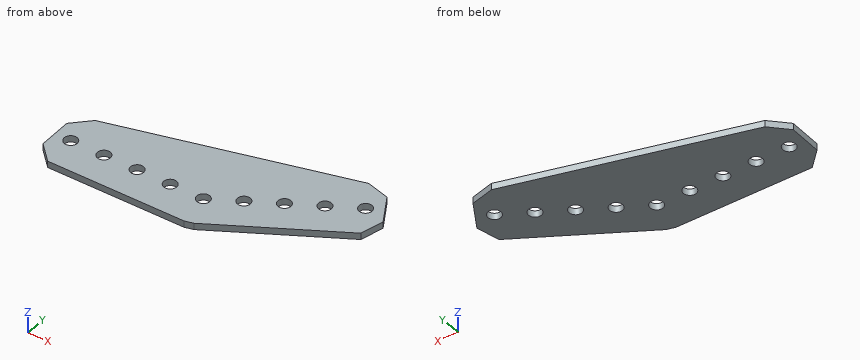
from build123d import *

# Parameters (mm, degrees)
SKETCH1_R           = 2.5
BOSS_EXTRUDE1_DEPTH = 2.5


with BuildPart() as part:
    # Sketch1 → Boss-Extrude1 (new body)
    with BuildSketch(Plane(origin=(0, 0, -1.25), x_dir=(-1, 0, 0), z_dir=(0, 0, -1))):
        Polygon((50.546, 12.7), (-37.42412006, 36.271522628), (-46.098381374, 33.947261314), (-52.448381374, 22.948738686), (-50.12412006, 14.274477372), (-4.902017026, -11.834515988), (-1.671986719, -12.7), (50.546, -12.7), (56.896, -6.35), (56.896, 6.35), align=None)
        with Locations((12.7, 0)):
            Circle(SKETCH1_R, mode=Mode.SUBTRACT)
        with Locations((25.4, 0)):
            Circle(SKETCH1_R, mode=Mode.SUBTRACT)
        Circle(SKETCH1_R, mode=Mode.SUBTRACT)
        with Locations((50.8, 0)):
            Circle(SKETCH1_R, mode=Mode.SUBTRACT)
        with Locations((38.1, 0)):
            Circle(SKETCH1_R, mode=Mode.SUBTRACT)
        with Locations((-43.994090512, 25.4)):
            Circle(SKETCH1_R, mode=Mode.SUBTRACT)
        with Locations((-32.995567884, 19.05)):
            Circle(SKETCH1_R, mode=Mode.SUBTRACT)
        with Locations((-21.997045256, 12.7)):
            Circle(SKETCH1_R, mode=Mode.SUBTRACT)
        with Locations((-10.998522628, 6.35)):
            Circle(SKETCH1_R, mode=Mode.SUBTRACT)
    extrude(amount=-BOSS_EXTRUDE1_DEPTH)


solid = part.part
The model under review builds one solid part; all positions refer to its coordinate system, in mm. Give positions to 0.01 mm unless a question says otherwise; leave off trailing zeros. Write each loop counter-clockwise with the first axis right and the second up, starting at its lowest first coordinate (ties: lowest second). Pieces come first, ordered by that corner, then holes.
1. Add section D-D, the plane y = 19.05. Write out the cut boundary in (x, z), plus the area to 3 significant figures.
2. For P1, Ø4.5, axis at x = 22, y = 12.7, coming from the +Z side, flat-tipped, find the tip position at first contact; note if it passes through.
3. Wall thickness on L1, parallel to Y at x = -12.5, z = 0; L2, parallel to Y at x = -50.8, z = 0.3; L3, parallel to Y at x = -22, z = 0.2: over which ranges is each line inside the solid? List them lowest first.
4. Add section A-A, the plane y = 0. Write out the cut boundary in (x, z).
5. Add section C-C, the plane x = -12.7. Write out the cut boundary in (y, z), plus the area to 3 significant figures.
6. Add section B-B, the plane z = -0.55. Count the separate pieces of the cut face and the enclosed holes in it, plus the area to 3 significant figures.
Worked answers:
1. outline: (-26.85, -1.25) - (30.5, -1.25) - (30.5, 1.25) - (-26.85, 1.25) - close; (35.5, -1.25) - (51.4, -1.25) - (51.4, 1.25) - (35.5, 1.25) - close
1. area: 183 mm2
2. P1: passes through
3. L1: y = -12.7 to -2.49, 2.49 to 22.89
3. L2: y = -12.45 to -2.5, 2.5 to 12.45
3. L3: y = -12.7 to 20.35
4. outline: (-56.9, -1.25) - (-53.3, -1.25) - (-53.3, 1.25) - (-56.9, 1.25) - close; (-48.3, -1.25) - (-40.6, -1.25) - (-40.6, 1.25) - (-48.3, 1.25) - close; (-35.6, -1.25) - (-27.9, -1.25) - (-27.9, 1.25) - (-35.6, 1.25) - close; (-22.9, -1.25) - (-15.2, -1.25) - (-15.2, 1.25) - (-22.9, 1.25) - close; (-10.2, -1.25) - (-2.5, -1.25) - (-2.5, 1.25) - (-10.2, 1.25) - close; (2.5, -1.25) - (25.4, -1.25) - (25.4, 1.25) - (2.5, 1.25) - close
5. outline: (-12.7, -1.25) - (-2.5, -1.25) - (-2.5, 1.25) - (-12.7, 1.25) - close; (2.5, -1.25) - (22.84, -1.25) - (22.84, 1.25) - (2.5, 1.25) - close
5. area: 76.4 mm2
6. separate pieces: 1
6. enclosed holes: 9
6. area: 3,190 mm2
